Verification items for the finished model (mm, model axes). A direction names the side the tool comes from. Give positions to 0.01 mm unless a question says otherwise; leave off trailing zeros. Loops run counter-clockwise (first coordinate to the right, second up) from the corner with the lowest first, then second, coordinate; pieces in that order, holes last. Notation, with made-up numbers: M 24,73 L 53,73 A36 cw 53,112 Z; hole C 35.25,8.25 d10. An arc over 180 degrees is marked long. Use a Markdown table: item, result.
from build123d import *

# Parameters (mm, degrees)
SKETCH1_R           = 2.55
SKETCH1_R_2         = 3.6
BOSS_EXTRUDE1_DEPTH = 3
FILLET1_R           = 0.5


with BuildPart() as part:
    # Sketch1 → Boss-Extrude1 (new body)
    with BuildSketch(Plane(origin=(0, 0, 0), x_dir=(1, 0, 0), z_dir=(0, 1, 0))):
        with BuildLine():
            Line((29.5, 32), (-29.5, 32))
            ThreePointArc((-29.5, 32), (-31.267766953, 31.267766953), (-32, 29.5))
            Line((-32, 29.5), (-32, -29.5))
            ThreePointArc((-32, -29.5), (-31.267766953, -31.267766953), (-29.5, -32))
            Line((-29.5, -32), (29.5, -32))
            ThreePointArc((29.5, -32), (31.267766953, -31.267766953), (32, -29.5))
            Line((32, -29.5), (32, 29.5))
            ThreePointArc((32, 29.5), (31.267766953, 31.267766953), (29.5, 32))
        make_face()
        with Locations((-10.25, 0.25)):
            Circle(SKETCH1_R, mode=Mode.SUBTRACT)
        with Locations((19.6, 0.25)):
            Circle(SKETCH1_R_2, mode=Mode.SUBTRACT)
        with Locations((19.6, 10.25)):
            Circle(SKETCH1_R, mode=Mode.SUBTRACT)
        with Locations((-0.25, 10.25)):
            Circle(SKETCH1_R, mode=Mode.SUBTRACT)
        with Locations((19.6, -19.75)):
            Circle(SKETCH1_R_2, mode=Mode.SUBTRACT)
        with Locations((-0.25, -9.75)):
            Circle(SKETCH1_R, mode=Mode.SUBTRACT)
        with Locations((19.6, -9.75)):
            Circle(SKETCH1_R, mode=Mode.SUBTRACT)
        with Locations((9.75, 0.25)):
            Circle(SKETCH1_R, mode=Mode.SUBTRACT)
        with Locations((-0.25, 0.25)):
            Circle(SKETCH1_R, mode=Mode.SUBTRACT)
        with Locations((-20.1, -19.75)):
            Circle(SKETCH1_R, mode=Mode.SUBTRACT)
        with Locations((-20.1, -9.75)):
            Circle(SKETCH1_R, mode=Mode.SUBTRACT)
        with Locations((-20.1, 0.25)):
            Circle(SKETCH1_R, mode=Mode.SUBTRACT)
        with Locations((-20.1, 10.25)):
            Circle(SKETCH1_R, mode=Mode.SUBTRACT)
        with Locations((19.6, 20.25)):
            Circle(SKETCH1_R_2, mode=Mode.SUBTRACT)
        with Locations((-20.1, 20.25)):
            Circle(SKETCH1_R, mode=Mode.SUBTRACT)
        with Locations((-0.25, -19.75)):
            Circle(SKETCH1_R, mode=Mode.SUBTRACT)
        with Locations((-0.25, 20.25)):
            Circle(SKETCH1_R, mode=Mode.SUBTRACT)
        with BuildLine():
            Line((3, 26.45), (-3.500000052, 26.45))
            ThreePointArc((-3.500000052, 26.45), (-5.000000052, 27.95), (-3.500000052, 29.45))
            Line((-3.500000052, 29.45), (3, 29.45))
            ThreePointArc((3, 29.45), (4.5, 27.95), (3, 26.45))
        make_face(mode=Mode.SUBTRACT)
        with BuildLine():
            Line((-23.649999471, 29.45), (-17.15, 29.45))
            ThreePointArc((-17.15, 29.45), (-15.65, 27.95), (-17.15, 26.45))
            Line((-17.15, 26.45), (-23.649999471, 26.45))
            ThreePointArc((-23.649999471, 26.45), (-25.149999471, 27.95), (-23.649999471, 29.45))
        make_face(mode=Mode.SUBTRACT)
        with BuildLine():
            Line((16.649999628, 29.45), (23.15, 29.45))
            ThreePointArc((23.15, 29.45), (24.65, 27.95), (23.15, 26.45))
            Line((23.15, 26.45), (16.649999628, 26.45))
            ThreePointArc((16.649999628, 26.45), (15.149999628, 27.95), (16.649999628, 29.45))
        make_face(mode=Mode.SUBTRACT)
        with BuildLine():
            Line((-17.15, -28.95), (-23.649999471, -28.95))
            ThreePointArc((-23.649999471, -28.95), (-25.149999471, -27.45), (-23.649999471, -25.95))
            Line((-23.649999471, -25.95), (-17.15, -25.95))
            ThreePointArc((-17.15, -25.95), (-15.65, -27.45), (-17.15, -28.95))
        make_face(mode=Mode.SUBTRACT)
        with BuildLine():
            Line((-3.500000052, -25.95), (3, -25.95))
            ThreePointArc((3, -25.95), (4.5, -27.45), (3, -28.95))
            Line((3, -28.95), (-3.500000052, -28.95))
            ThreePointArc((-3.500000052, -28.95), (-5.000000052, -27.45), (-3.500000052, -25.95))
        make_face(mode=Mode.SUBTRACT)
        with BuildLine():
            Line((23.15, -28.95), (16.649999628, -28.95))
            ThreePointArc((16.649999628, -28.95), (15.149999628, -27.45), (16.649999628, -25.95))
            Line((16.649999628, -25.95), (23.15, -25.95))
            ThreePointArc((23.15, -25.95), (24.65, -27.45), (23.15, -28.95))
        make_face(mode=Mode.SUBTRACT)
    extrude(amount=BOSS_EXTRUDE1_DEPTH)

    # Fillet1
    fillet1_edges = [part.edges().sort_by_distance(p)[0] for p in [
        (-32, 0, 0),
        (-31.267766953, 0, -31.267766953),
        (0, 0, -32),
        (31.267766953, 0, -31.267766953),
        (-31.267766953, 3, -31.267766953),
        (-32, 3, 0),
        (-31.267766953, 3, 31.267766953),
        (0, 3, 32),
        (31.267766953, 3, 31.267766953),
        (32, 3, 0),
        (31.267766953, 3, -31.267766953),
        (32, 0, 0),
        (0, 3, -32),
        (31.267766953, 0, 31.267766953),
        (0, 0, 32),
        (-31.267766953, 0, 31.267766953),
    ]]
    fillet(fillet1_edges, radius=FILLET1_R)


solid = part.part
(1) Cross-section at C-C on z = -20.25. Record the cut outline in (x, y), then the cut area to 3 significant figures.
Results below:
| item | result |
|---|---|
| outline | M -32,0.5 A0.5 ccw -31.5,0 L -22.65,0 L -22.65,3 L -31.5,3 A0.5 ccw -32,2.5 Z; M -17.55,0 L -2.8,0 L -2.8,3 L -17.55,3 Z; M 2.3,0 L 16,0 L 16,3 L 2.3,3 Z; M 23.2,0 L 31.5,0 A0.5 ccw 32,0.5 L 32,2.5 A0.5 ccw 31.5,3 L 23.2,3 Z |
| area | 140 mm^2 |
(2) Material ranges on line 1 (X direction, y = 1.55, z = 9.75); line 2 (X direction, y = 1.7, z = -0.25); line 3 (X direction, y = 1.3, z = -20.25), recorded low to high.
Results below:
| item | result |
|---|---|
| line 1 | -32 to -22.65, -17.55 to -2.8, 2.3 to 17.05, 22.15 to 32 |
| line 2 | -32 to -22.65, -17.55 to -12.8, -7.7 to -2.8, 2.3 to 7.2, 12.3 to 16, 23.2 to 32 |
| line 3 | -32 to -22.65, -17.55 to -2.8, 2.3 to 16, 23.2 to 32 |
(3) Draft check along X on faces 1 (the cylindrical face through (-0.8, 1.48, 12.24)), 2 (the cylindrical face through (-31.287, 1.486, 31.248)), 3 (the flat face through (0, 3, -7)). Enter one of: +X half, -X half, draft (parallel to the pull), parting line (faces both ways), or undercut.
Results below:
| item | result |
|---|---|
| face 1 | undercut |
| face 2 | -X half |
| face 3 | draft |
(4) Cross-section at A-A on z = 27.45. Record the cut outline in (x, y), then the cut area to 3 significant figures.
Results below:
| item | result |
|---|---|
| outline | M -32,0.5 A0.5 ccw -31.5,0 L -25.15,0 L -25.15,3 L -31.5,3 A0.5 ccw -32,2.5 Z; M -15.65,0 L -5,0 L -5,3 L -15.65,3 Z; M 4.5,0 L 15.15,0 L 15.15,3 L 4.5,3 Z; M 24.65,0 L 31.5,0 A0.5 ccw 32,0.5 L 32,2.5 A0.5 ccw 31.5,3 L 24.65,3 Z |
| area | 106 mm^2 |
(5) Cross-section at B-B on x = -10.25. Record the cut outline in (y, z), then the cut area to 3 significant figures.
Results below:
| item | result |
|---|---|
| outline | M 0,-31.5 A0.5 ccw 0.5,-32 L 2.5,-32 A0.5 ccw 3,-31.5 L 3,-2.8 L 0,-2.8 Z; M 0,2.3 L 3,2.3 L 3,31.5 A0.5 ccw 2.5,32 L 0.5,32 A0.5 ccw 0,31.5 Z |
| area | 176 mm^2 |
(6) Set-up check for faces 4 (the flat face through (-20, 1, -26.45)), 5 (the flat face through (-32, 1, 0)): record each of +Z, -Z, +X, -X, +Y, -Y from which the full face is reachable in a straight line by a thin tool's end or side.
Results below:
| item | result |
|---|---|
| face 4 | +Y, -Y |
| face 5 | +Z, -Z, -X, +Y, -Y |
(7) Cross-section at D-D on x = 9. Record the cut outline in (y, z), then the cut area to 3 significant figures.
Results below:
| item | result |
|---|---|
| outline | M 0,-31.5 A0.5 ccw 0.5,-32 L 2.5,-32 A0.5 ccw 3,-31.5 L 3,-2.69 L 0,-2.69 Z; M 0,2.19 L 3,2.19 L 3,31.5 A0.5 ccw 2.5,32 L 0.5,32 A0.5 ccw 0,31.5 Z |
| area | 177 mm^2 |
